For this review, take the finished solid that the model builds, in its own axes (mm). A direction names the side the tool comes from. Give positions to 0.01 mm unless a question says otherwise; leave off trailing zeros. Loops run counter-clockwise (first coordinate to the right, second up) from the corner with the lowest first, then second, coordinate; pieces in that order, holes last.
```python
from build123d import *

# Parameters (mm, degrees)
PAD_DEPTH = 6


with BuildPart() as part:
    # Sketch → Pad (new body)
    with BuildSketch(Plane.XY):
        Polygon((9.814955, 0), (4.907477, 8.5), (-4.907477, 8.5), (-9.814955, 0), (-4.907477, -8.5), (4.907477, -8.5), align=None)
        Polygon((7.505553, 0), (3.752777, 6.5), (-3.752777, 6.5), (-7.505553, 0), (-3.752777, -6.5), (3.752777, -6.5), align=None, mode=Mode.SUBTRACT)
    extrude(amount=PAD_DEPTH)


solid = part.part
```
Q1. Machinability: for faces 1 (the flat face through (0, 8.5, 3)), 2 (the flat face through (0, 6.5, 3)), which of the approach directions +Z, -Z, +X, -X, +Y, -Y give a long, thin tool a straight path to every point of the face, cutting with its end or side? Answer none if there is none.
Answers:
face 1: +Z, -Z, +X, -X, +Y
face 2: +Z, -Z
Q2. Mouldability with a two-part tool opening along Y and no side actions: class faces 3 (the flat face through (7.396, 4.19, 2.958)), 4 (the flat face through (7.327, -4.31, 2.958)), 5 (the flat face through (5.6, -3.3, 3)), 6 (the flat face through (-5.66, -3.2, 2.96)) as +Y half, -Y half, draft (parallel to the pull), parting line (faces both ways), or undercut.
Answers:
face 3: +Y half
face 4: -Y half
face 5: undercut
face 6: undercut
Q3. Consider section D-D on x = 8.5. Give the boundary of the cut face in (y, z).
Answers:
outline: (-2.28, 0) - (2.28, 0) - (2.28, 6) - (-2.28, 6) - close
Q4. For probe 1 along Y at (x, z) = (2.25, 1.95); probe 2 along X at (y, z) = (-6.25, 5.4); probe 3 along Y at (x, z) = (7, 3.2), list the stretches that pass through material, from the lowest coordinate up.
Answers:
probe 1: y = -8.5 to -6.5, 6.5 to 8.5
probe 2: x = -6.21 to -3.9, 3.9 to 6.21
probe 3: y = -4.88 to -0.88, 0.88 to 4.88
Q5. Consider section B-B on z = 1.45. Give the boundary of the cut face in (x, y), plus the area to 3 significant figures.
Answers:
outline: (-9.81, 0) - (-4.91, -8.5) - (4.91, -8.5) - (9.81, 0) - (4.91, 8.5) - (-4.91, 8.5) - close; hole (-7.51, 0) - (-3.75, -6.5) - (3.75, -6.5) - (7.51, 0) - (3.75, 6.5) - (-3.75, 6.5) - close
area: 104 mm2
Q6. For pin 1 Ø1 at (x, z) = (-6.5, 2.5) entering from -Y; pin 2 Ø1 at (y, z) = (-1, 1) entering from +X, all flat-tipped, find the tip position at first contact; note any pin that passes through.
Answers:
pin 1: stops at y = -6.61
pin 2: stops at x = 9.53
Q7. Consider section C-C on y = -4.25. Give the boundary of the cut face in (x, z).
Answers:
outline: (-7.36, 0) - (-5.05, 0) - (-5.05, 6) - (-7.36, 6) - close; (5.05, 0) - (7.36, 0) - (7.36, 6) - (5.05, 6) - close
Q8. Consider section A-A on x = -3. Give the boundary of the cut face in (y, z).
Answers:
outline: (-8.5, 0) - (-6.5, 0) - (-6.5, 6) - (-8.5, 6) - close; (6.5, 0) - (8.5, 0) - (8.5, 6) - (6.5, 6) - close
